Design review of the part built by this model. Coordinates are the model's own, in mm. A direction names the side the tool comes from. Round coordinates to 2 decimals unless told otherwise and drop trailing zeros. Order: outer loops, then holes, each group sorted by start corner. A loop starts at its lowest first (then second) coordinate and runs counter-clockwise, first axis right, second up. Notation, with made-up numbers: M 25,29.25 L 35,29.25 A27 cw 35,59.25 Z; hole C 43.5,-20 d10. An arc over 180 degrees is marked long. Use a Markdown table: item, result. Add a question column.
(1) Take a section at C-C (x = 9). Write out the cut boundary in (y, z), then the cut area to 3 significant figures.
(2) Take a section at B-B (z = -7). Write out the cut boundary in (x, y).
(3) Machinability: for faces 5 (the face through (7.46, 83.52, -2.05)), 6 (the face through (2.335, 8.173, -8.493)), which of the approach directions +Z, -Z, +X, -X, +Y, -Y give a long, thin tool a straight path to every point of the face, cutting with its end or side? Answer none if there is none.
(4) For pin 1 (5 mm diameter, centred on x = 21.91, y = 6.36, fed in from +Z), flat-tipped, find the tip position at first contact; note if it passes through.
(5) Take a section at A-A (x = 12.7). Write out the cut boundary in (y, z).
(6) The part is to be moulded in two halves that separate along X. For faces 1 (the face through (0, 44, -6)), 2 (the face through (17.94, 83.81, -2.05)), 3 (the face through (13, 0, -6)), 4 (the face through (19.854, 7.005, -8.493)), say which applies: released by +X, released by -X, zero draft, split by the parting line, or undercut.
(7) To check wall thickness, follow probe 1 along Y at (x, z) = (3.5, -6); probe 2 along Y at (x, z) = (5.5, -1.5); probe 3 along Y at (x, z) = (12.75, -5.75). State the ranges of each line that lie inside material, in increasing order. Write a range as from..to.
```python
from build123d import *

# Parameters (mm, degrees)
SKETCH1_W                                      = 25.4
SKETCH1_H                                      = 12.7
BOSS_EXTRUDE1_DEPTH                            = 90.0176
CBORE_FOR_8_SOCKET_HEAD_CAP_SCREW1_D           = 4.3053
CBORE_FOR_8_SOCKET_HEAD_CAP_SCREW1_DEPTH       = 19.05
CBORE_FOR_8_SOCKET_HEAD_CAP_SCREW1_CBORE_D     = 7.9375
CBORE_FOR_8_SOCKET_HEAD_CAP_SCREW1_CBORE_DEPTH = 4.1656
CBORE_FOR_8_SOCKET_HEAD_CAP_SCREW1_TIP         = 1.293442612
F_1_2_0_5_DIAMETER_HOLE1_D                     = 12.7
F_1_2_0_5_DIAMETER_HOLE1_DEPTH                 = 15.24
F_1_2_0_5_DIAMETER_HOLE1_TIP                   = 3.815464931


with BuildPart() as part:
    # Sketch1 → Boss-Extrude1 (new body)
    with BuildSketch(Plane(origin=(0, 0, 0), x_dir=(1, 0, 0), z_dir=(0, 1, 0))):
        with Locations((12.7, 6.35)):
            Rectangle(SKETCH1_W, SKETCH1_H)
    extrude(amount=BOSS_EXTRUDE1_DEPTH)

    # CBORE for #8 Socket Head Cap Screw1
    with Locations(Plane(origin=(3.4925, 6.357975427, 0), x_dir=(1, 0, 0), z_dir=(0, 0, 1))):
        with Locations((0, 0), (18.415, 0), (18.415, 77.309624573), (0, 77.309624573)):
            CounterBoreHole(CBORE_FOR_8_SOCKET_HEAD_CAP_SCREW1_D / 2, CBORE_FOR_8_SOCKET_HEAD_CAP_SCREW1_CBORE_D / 2, CBORE_FOR_8_SOCKET_HEAD_CAP_SCREW1_CBORE_DEPTH, depth=CBORE_FOR_8_SOCKET_HEAD_CAP_SCREW1_DEPTH)
            with Locations((0, 0, -(CBORE_FOR_8_SOCKET_HEAD_CAP_SCREW1_DEPTH + CBORE_FOR_8_SOCKET_HEAD_CAP_SCREW1_TIP / 2))):  # 118° drill point
                Cone(0, CBORE_FOR_8_SOCKET_HEAD_CAP_SCREW1_D / 2, CBORE_FOR_8_SOCKET_HEAD_CAP_SCREW1_TIP, mode=Mode.SUBTRACT)

    # 1/2 (0.5) Diameter Hole1
    with Locations(Plane(origin=(12.7, 45.012787713, 0), x_dir=(1, 0, 0), z_dir=(0, 0, 1))):
        with Locations((0, 0)):
            Hole(F_1_2_0_5_DIAMETER_HOLE1_D / 2, depth=F_1_2_0_5_DIAMETER_HOLE1_DEPTH)
            with Locations((0, 0, -(F_1_2_0_5_DIAMETER_HOLE1_DEPTH + F_1_2_0_5_DIAMETER_HOLE1_TIP / 2))):  # 118° drill point
                Cone(0, F_1_2_0_5_DIAMETER_HOLE1_D / 2, F_1_2_0_5_DIAMETER_HOLE1_TIP, mode=Mode.SUBTRACT)


solid = part.part
```
Verdict:
| question | item | result |
|---|---|---|
| 1 | outline | M 0,-12.7 L 39.85,-12.7 L 39.85,0 L 0,0 Z; M 50.17,-12.7 L 90.02,-12.7 L 90.02,0 L 50.17,0 Z |
| 1 | area | 1,010 mm^2 |
| 2 | outline | M 0,0 L 25.4,0 L 25.4,90.02 L 0,90.02 Z; hole C 3.49,6.36 d4.31; hole C 3.49,83.67 d4.31; hole C 12.7,45.01 d12.7; hole C 21.91,6.36 d4.31; hole C 21.91,83.67 d4.31 |
| 3 | face 5 | +Z |
| 3 | face 6 | +Z, -Z |
| 4 | pin 1 | stops at z = -4.17 |
| 5 | outline | M 0,-12.7 L 38.66,-12.7 L 38.66,0 L 0,0 Z; M 51.36,-12.7 L 90.02,-12.7 L 90.02,0 L 51.36,0 Z |
| 6 | face 1 | released by -X |
| 6 | face 2 | undercut |
| 6 | face 3 | zero draft |
| 6 | face 4 | undercut |
| 7 | probe 1 | y = 0..4.21, 8.51..81.51, 85.82..90.02 |
| 7 | probe 2 | y = 0..2.93, 9.78..80.24, 87.09..90.02 |
| 7 | probe 3 | y = 0..38.66, 51.36..90.02 |
